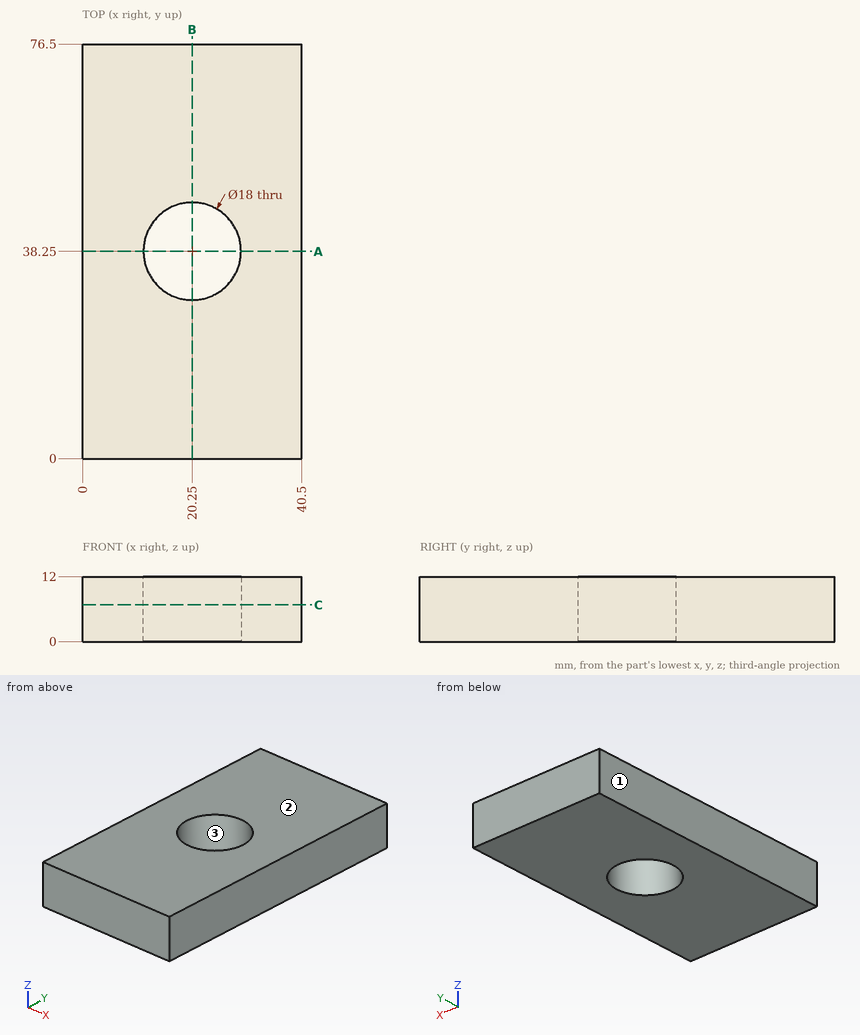
Check sheet for the drawn part. Datum: minimum x, y, z corner. Units: mm. Round coordinates to 2 decimals unless told otherwise and drop trailing zeros. Write each loop counter-clockwise with the first axis right and the second up, starting at its lowest first coordinate (ties: lowest second). Pieces come first, ordered by that corner, then holes. Notation, with made-up numbers: (54, 23.25) -> (69, 23.25) arc R24 cw to (69, 39.25) -> close; hole circle Ø9 at (-4.5, 42.5). An arc over 180 degrees is marked (long way). One line per item, written item: value. Start each with the question number.
(1) Cross-section at A-A, the plane y = 38.25. Record the cut outline in (x, z), and give its area (3 significant figures).
(2) Go/stop test with a flat-tipped pin: pin 1 Ø2 at (x, z) = (31, 7) entering from -Y. Record where the tip stops, or that it passes through.
(3) Scan lines: line 1 (Y direction, x = 20.25, z = 3); line 2 (X direction, y = 38.5, z = 7.5); line 3 (Y direction, x = 12, z = 11.25). Record each from-to range of solid material in increasing order. Write a range as [from, to].
(4) Cross-section at B-B, the plane x = 20.25. Record the cut outline in (y, z), and give its area (3 significant figures).
(5) Draft check along X on the marked faces 1, 2 and 3. Enter one of: +X half, -X half, draft (parallel to the pull), parting line (faces both ways), or undercut.
(6) Cross-section at C-C, the plane z = 6.75. Record the cut outline in (x, y).
Answer:
1. outline: (0, 0) -> (11.25, 0) -> (11.25, 12) -> (0, 12) -> close; (29.25, 0) -> (40.5, 0) -> (40.5, 12) -> (29.25, 12) -> close
1. area: 270 mm²
2. pin 1: y = 0
3. line 1: [0, 29.25], [47.25, 76.5]
3. line 2: [0, 11.25], [29.25, 40.5]
3. line 3: [0, 34.65], [41.85, 76.5]
4. outline: (0, 0) -> (29.25, 0) -> (29.25, 12) -> (0, 12) -> close; (47.25, 0) -> (76.5, 0) -> (76.5, 12) -> (47.25, 12) -> close
4. area: 702 mm²
5. face 1: -X half
5. face 2: draft
5. face 3: undercut
6. outline: (0, 0) -> (40.5, 0) -> (40.5, 76.5) -> (0, 76.5) -> close; hole circle Ø18 at (20.25, 38.25)
